```python
from build123d import *

# Parameters (mm, degrees)
SKETCH_1_R          = 27
EXTRUDE_1_DEPTH     = 2
EXTRUDE_2_DEPTH     = 20
SKETCH_3_R          = 2.5
EXTRUDE_3_DEPTH     = 20
SKETCH_4_R          = 1
CUT_EXTRUDE_1_DEPTH = 15


with BuildPart() as part:
    # 草图1 → 凸台-拉伸1 (new body)
    with BuildSketch(Plane.XY):
        Circle(SKETCH_1_R)
    extrude(amount=EXTRUDE_1_DEPTH)

    # 草图2 → 凸台-拉伸2 (add)
    with BuildSketch(Plane.XY):
        Polygon((-2.5, 0), (-14.5, 6.92820323), (-24.5, 6.92820323), (-24.5, 5.92820323), (-14.767949192, 5.92820323), (-3, -0.866025404), align=None)
        Polygon((-12.425136654, 22.223095625), (-13.132243435, 21.515988843), (-6.250644314, 14.634389723), (-2.733692779, 1.508947908), (-1.767766953, 1.767766953), (-5.354068842, 15.152027813), align=None)
        Polygon((6.92820323, 24.5), (5.92820323, 24.5), (5.92820323, 14.767949192), (-0.866025404, 3), (0, 2.5), (6.92820323, 14.5), align=None)
        Polygon((22.223095625, 12.425136654), (21.515988843, 13.132243435), (14.634389723, 6.250644314), (1.508947908, 2.733692779), (1.767766953, 1.767766953), (15.152027813, 5.354068842), align=None)
        Polygon((24.5, -6.92820323), (24.5, -5.92820323), (14.767949192, -5.92820323), (3, 0.866025404), (2.5, 0), (14.5, -6.92820323), align=None)
        Polygon((12.425136654, -22.223095625), (13.132243435, -21.515988843), (6.250644314, -14.634389723), (2.733692779, -1.508947908), (1.767766953, -1.767766953), (5.354068842, -15.152027813), align=None)
        Polygon((-6.92820323, -24.5), (-5.92820323, -24.5), (-5.92820323, -14.767949192), (0.866025404, -3), (0, -2.5), (-6.92820323, -14.5), align=None)
        Polygon((-22.223095625, -12.425136654), (-21.515988843, -13.132243435), (-14.634389723, -6.250644314), (-1.508947908, -2.733692779), (-1.767766953, -1.767766953), (-15.152027813, -5.354068842), align=None)
    extrude(amount=-EXTRUDE_2_DEPTH)

    # 草图3 → 凸台-拉伸3 (add)
    with BuildSketch(Plane.XY.offset(2)):
        Circle(SKETCH_3_R)
    extrude(amount=EXTRUDE_3_DEPTH)

    # 草图4 → 切除-拉伸1 (cut)
    with BuildSketch(Plane.XY.offset(22)):
        Circle(SKETCH_4_R)
    extrude(amount=-CUT_EXTRUDE_1_DEPTH, mode=Mode.SUBTRACT)


solid = part.part
```
Can you work these out from the model? Positions are in its coordinate system, mm. A direction names the side the tool comes from. Coordinates: 2 decimals unless noted, no trailing zeros. Loops run counter-clockwise (first coordinate to the right, second up) from the corner with the lowest first, then second, coordinate; pieces in that order, holes last. Notation, with made-up numbers: (-12.75, -8.5) - (44.25, -8.5) arc R24 ccw to (44.25, 25.5) - close; hole circle Ø4 at (19.5, 12). An arc over 180 degrees is marked (long way). Answer as CSV lines item,"result". Start each with the question number.
1) I need wall thicknesses on line 1 (Y direction, x = 0, z = 12); line 2 (X direction, y = 9, z = -12.5); line 3 (Z direction, x = 14, y = -14). Which ranges of each line are inside material? Lowest first, please. Write a range as from..to.
2) Suppose I cut it at D-D (y = 18). Please give me the cut outline in (x, z), plus the area to 3 significant figures.
3) Suppose I cut it at A-A (z = 17). Please give me the cut outline in (x, y), plus the area to 3 significant figures.
4) For pin 1 (12 mm diameter, centred on x = 13, z = 3, fed in from -Y); pin 2 (6 mm diameter, centred on x = -16, z = -10, fed in from -Y); pin 3 (1.1 mm diameter, centred on y = -6.5, z = -12, fed in from +X); pin 4 (4 mm diameter, centred on x = -19.5, z = 4.5, fed in from +Y), each with a flat end and sliding along its axis, tell me the tip position at first contact or that it passes through.
5) Thinking about a two-plate mould opening in Y: for faces 4 (the flat face through (8.366, 3.536, -9.86)), 5 (the flat face through (3.536, -8.366, -9.86)), 6 (the flat face through (1, -1, 22)), which applies, pulls with the +Y half, pulls with the -Y half, needs draft (parallel to the pull), parting line crosses it, or undercut?
6) Which directions (+Z, -Z, +X, -X, +Y, -Y) give clear straight access to the entire face, cutting with the end or side of a thin tool? Please do faces 1 (the flat face through (-20, 5.928, -10)), 2 (the flat face through (-2.6, -9, -9.9)), 3 (the flat face through (18.6, 8.8, -9.9)).
7) Suppose I cut it at B-B (z = -8). Count the separate pieces of the cut face and the enclosed holes in it, plus the area to 3 significant figures.
8) Suppose I cut it at C-C (x = 11). Please give me the cut outline in (y, z).
Check result:
1,line 1,"y = -2.5..-1, 1..2.5"
1,line 2,"x = -4.74..-3.71, 2.6..3.75, 17.38..18.8"
1,line 3,"z = 0..2"
2,outline,"(-20.12, 0) - (-9.62, 0) - (-9.62, -20) - (-8.2, -20) - (-8.2, 0) - (5.93, 0) - (5.93, -20) - (6.93, -20) - (6.93, 0) - (20.12, 0) - (20.12, 2) - (-20.12, 2) - close"
2,area,"129 mm²"
3,outline,"circle Ø5 at (0, 0); hole circle Ø2 at (0, 0)"
3,area,"16.5 mm²"
4,pin 1,"stops at y = -26.05"
4,pin 2,"stops at y = -10.62"
4,pin 3,"stops at x = 24.5"
4,pin 4,"passes through"
5,face 4,"undercut"
5,face 5,"pulls with the -Y half"
5,face 6,"needs draft"
6,face 1,"-Z, -X"
6,face 2,"-Z, -Y"
6,face 3,"-Z, +X"
7,separate pieces,"8"
7,enclosed holes,"0"
7,area,"189 mm²"
8,outline,"(-24.66, 0) - (-20.8, 0) - (-20.8, -20) - (-19.38, -20) - (-19.38, 0) - (-4.91, 0) - (-4.91, -20) - (-3.75, -20) - (-3.75, 0) - (4.24, 0) - (4.24, -20) - (5.28, -20) - (5.28, 0) - (24.66, 0) - (24.66, 2) - (-24.66, 2) - close"
